Part model, mm, in its own coordinate system. A direction names the side the tool comes from. Coordinates: 2 decimals unless noted, no trailing zeros. Write each loop counter-clockwise with the first axis right and the second up, starting at its lowest first coordinate (ties: lowest second). Pieces come first, ordered by that corner, then holes. Notation, with made-up numbers: (-22, -32.75) - (9, -32.75) arc R19 ccw to (9, -6.75) - close; hole circle Ø2 at (76.25, 51.5). An arc over 180 degrees is marked (long way). Use a Markdown table: item, result.
```python
from build123d import *

# Parameters (mm, degrees)
SKETCH4_W           = 50.8
SKETCH4_H           = 38.1
BOSS_EXTRUDE3_DEPTH = 127
SKETCH2_W           = 127
SKETCH2_H           = 38.1
BOSS_EXTRUDE2_DEPTH = 19.05


with BuildPart() as part:
    # Sketch1 → Revolve1 (revolve)
    with BuildSketch(Plane.XY):
        with BuildLine():
            Line((50.8, 0), (50.8, -660.4))
            Line((50.8, -660.4), (9.120840186, -901.7))
            Line((9.120840186, -901.7), (0, -914.4))
            Line((0, -914.4), (0, 50.8))
            ThreePointArc((0, 50.8), (35.921024484, 35.921024484), (50.8, 0))
        make_face()
    revolve(axis=Axis((0, -914.4, 0), (0, 1, 0)))

    # Sketch4 → Boss-Extrude3 (add, symmetric)
    with BuildSketch(Plane.XY):
        with Locations((25.4, -19.05)):
            Rectangle(SKETCH4_W, SKETCH4_H)
    extrude(amount=BOSS_EXTRUDE3_DEPTH, both=True)

    # Sketch2 → Boss-Extrude2 (add, symmetric)
    with BuildSketch(Plane.XY):
        with Locations((63.5, -285.75)):
            Rectangle(SKETCH2_W, SKETCH2_H)
    extrude(amount=BOSS_EXTRUDE2_DEPTH, both=True)

    # Sketch5 → Cut-Revolve1 (revolve, cut)
    with BuildSketch(Plane.XY.offset(127)):
        with BuildLine():
            Line((50.8, 0), (50.8, -38.1))
            ThreePointArc((50.8, -38.1), (31.75, -19.05), (50.8, 0))
        make_face()
    cut_revolve1 = revolve(axis=Axis((50.8, 0, 127), (0, -1, 0)), mode=Mode.SUBTRACT)

    # Mirror1: Cut-Revolve1 across plane
    add(cut_revolve1.mirror(Plane.XY), mode=Mode.SUBTRACT)

    # Sketch6 → Cut-Revolve2 (revolve, cut)
    with BuildSketch(Plane.XY):
        with BuildLine():
            Line((127, -266.7), (127, -304.8))
            ThreePointArc((127, -304.8), (107.95, -285.75), (127, -266.7))
        make_face()
    revolve(axis=Axis((127, -266.7, 0), (0, -1, 0)), mode=Mode.SUBTRACT)


solid = part.part
```
Item 1: Two-plate mould, pull along X, no slides. Class faces 4 (the face through (-23.544, -782.739, 18.053)), 5 (the face through (50.8, -19, 2)), 6 (the face through (0, -19, -88)): pulls with the +X half, pulls with the -X half, needs draft (parallel to the pull), parting line crosses it, or undercut.
From the geometry:
| item | result |
|---|---|
| face 4 | parting line crosses it |
| face 5 | pulls with the +X half |
| face 6 | pulls with the -X half |
Item 2: Drop flat-ended pins along their axis: P1, Ø1.5, axis at x = 50.5, z = 59.5, coming from the +Y side; P2, Ø2, axis at y = -182.5, z = 29.5, coming from the -X side; P3, Ø19, axis at x = 103, z = -6, coming from the -Y side. Give the stop position or say it passes through.
From the geometry:
| item | result |
|---|---|
| P1 | y = 0 |
| P2 | x = -42.05 |
| P3 | y = -304.8 |
Item 3: Band-saw the part on B-B, the plane z = 87. Give the cut face in (x, y), then the cut area to 3 significant figures.
From the geometry:
| item | result |
|---|---|
| outline | (0, -38.1) - (50.8, -38.1) - (50.8, 0) - (0, 0) - close |
| area | 1,940 mm^2 |
Item 4: Which spindle directions (+Z, -Z, +X, -X, +Y, -Y) get a long thin tool onto all of the face, cutting with end or side? Do faces 1 (the face through (0, -19, 89)), 2 (the face through (25, 0, 79)), 3 (the face through (25, 0, -77)). Say none if no direction does.
From the geometry:
| item | result |
|---|---|
| face 1 | +Z, -X, +Y, -Y |
| face 2 | +Z, +X, +Y |
| face 3 | -Z, +X, +Y |
Item 5: Band-saw the part on A-A, the plane y = -453. Give the cut face in (x, z), then the cut area to 3 significant figures.
From the geometry:
| item | result |
|---|---|
| outline | circle Ø101.6 at (0, 0) |
| area | 8,110 mm^2 |
Item 6: Drill centre lines: probe 1 along Y at (x, z) = (89, -15.5); probe 2 along Y at (x, z) = (16.5, -87.5); probe 3 along Z at (x, y) = (115, -281). Where is each one in solid material? Low to high.
From the geometry:
| item | result |
|---|---|
| probe 1 | -304.8 to -266.7 |
| probe 2 | -38.1 to 0 |
| probe 3 | -19.05 to -14.01, 14.01 to 19.05 |
